Work out the finished part from the listing and answer in its coordinate system (mm). A direction names the side the tool comes from. Coordinates: 2 decimals unless noted, no trailing zeros. Use a Markdown table: item, result.
from build123d import *

# Parameters (mm, degrees)
SKIZZE2_W                            = 100
SKIZZE2_H                            = 39.364160046
AUFSATZ_LINEAR_AUSTRAGEN1_DEPTH      = 30
SCHNITT_LINEAR_AUSTRAGEN1_DEPTH      = 40
SCHNITT_LINEAR_AUSTRAGEN1_DEPTH_BACK = 40
SKIZZE10_R                           = 5
SKIZZE17_R                           = 1.4
SCHNITT_LINEAR_AUSTRAGEN2_DEPTH      = 103.710939516
SKIZZE24_R                           = 1.55
SCHNITT_LINEAR_AUSTRAGEN4_DEPTH      = 112.577493681
SKIZZE37_R                           = 0.736865544
SCHNITT_LINEAR_AUSTRAGEN9_DEPTH      = 112.577493681
SKIZZE40_R                           = 2.1
SCHNITT_LINEAR_AUSTRAGEN10_DEPTH     = 6
SKIZZE42_R                           = 0.75
SCHNITT_LINEAR_AUSTRAGEN12_DEPTH     = 10
VERRUNDUNG1_R                        = 1
SKIZZE46_R                           = 2.85
SCHNITT_LINEAR_AUSTRAGEN15_DEPTH     = 10
SCHNITT_LINEAR_START                 = -5
SCHNITT_LINEAR_AUSTRAGEN25_DEPTH     = 2.7
LINEARES_MUSTER1_COUNT               = 5
LINEARES_MUSTER1_PITCH               = 17
SPIEGELN2_COPY_1_SKETCH_R            = 2.85
SPIEGELN2_COPY_1_DEPTH               = 10
SPIEGELN2_COPY_2_SKETCH_R            = 2.85
SPIEGELN2_COPY_2_DEPTH               = 10
SPIEGELN2_COPY_3_SKETCH_R            = 2.85
SPIEGELN2_COPY_3_DEPTH               = 10
SPIEGELN2_COPY_4_SKETCH_R            = 2.85
SPIEGELN2_COPY_4_DEPTH               = 10
SPIEGELN2_START                      = -5
SPIEGELN2_COPY_5_DEPTH               = 2.7
SPIEGELN2_COPY_6_DEPTH               = 2.7
SPIEGELN2_COPY_7_DEPTH               = 2.7
SPIEGELN2_COPY_8_DEPTH               = 2.7
SKIZZE45_W                           = 15
SKIZZE45_H                           = 39.364160046
SCHNITT_LINEAR_AUSTRAGEN14_DEPTH     = 100


with BuildPart() as part:
    # Skizze2 → Aufsatz-Linear austragen1 (new body)
    with BuildSketch(Plane.XY):
        with Locations((50, 19.682080023)):
            Rectangle(SKIZZE2_W, SKIZZE2_H)
    extrude(amount=AUFSATZ_LINEAR_AUSTRAGEN1_DEPTH)

    # Skizze10 → Schnitt-Linear austragen1 (cut, two sides: drawn at the far end of the back side and taken through both)
    with BuildSketch(Plane.ZY.offset(-50).offset(-SCHNITT_LINEAR_AUSTRAGEN1_DEPTH_BACK)):
        with Locations((14.945770016, 20.027045739)):
            Circle(SKIZZE10_R)
    extrude(amount=SCHNITT_LINEAR_AUSTRAGEN1_DEPTH + SCHNITT_LINEAR_AUSTRAGEN1_DEPTH_BACK, mode=Mode.SUBTRACT)

    # Skizze17 → Schnitt-Linear austragen2 (cut, through all)
    with BuildSketch(Plane.ZY.offset(-90)):
        with Locations((14.945770016, 20.027045739)):
            Circle(SKIZZE17_R)
    schnitt_linear_austragen2 = extrude(amount=-SCHNITT_LINEAR_AUSTRAGEN2_DEPTH, mode=Mode.SUBTRACT)

    # Spiegeln1: Schnitt-Linear austragen2 across plane
    add(schnitt_linear_austragen2.mirror(Plane.ZY.offset(-50)), mode=Mode.SUBTRACT)

    # Skizze24 → Schnitt-Linear austragen4 (cut, through all)
    with BuildSketch(Plane.XY.offset(30)):
        with Locations((16, 31.364160046)):
            Circle(SKIZZE24_R)
        with Locations((33, 31.364160046)):
            Circle(SKIZZE24_R)
        with Locations((50, 31.364160046)):
            Circle(SKIZZE24_R)
        with Locations((67, 31.364160046)):
            Circle(SKIZZE24_R)
        with Locations((84, 31.364160046)):
            Circle(SKIZZE24_R)
    schnitt_linear_austragen4 = extrude(amount=-SCHNITT_LINEAR_AUSTRAGEN4_DEPTH, mode=Mode.SUBTRACT)

    # Skizze37 → Schnitt-Linear austragen9 (cut, through all)
    with BuildSketch(Plane(origin=(100, 0, 0), x_dir=(0, 0, -1), z_dir=(1, 0, 0))):
        with Locations((-18.924590299, 18.633559666)):
            Circle(SKIZZE37_R)
    extrude(amount=-SCHNITT_LINEAR_AUSTRAGEN9_DEPTH, mode=Mode.SUBTRACT)

    # Skizze40 → Schnitt-Linear austragen10 (cut)
    with BuildSketch(Plane(origin=(100, 0, 0), x_dir=(0, 0, -1), z_dir=(1, 0, 0))):
        with Locations((-18.924590299, 18.633559666)):
            Circle(SKIZZE40_R)
    extrude(amount=-SCHNITT_LINEAR_AUSTRAGEN10_DEPTH, mode=Mode.SUBTRACT)

    # Skizze42 → Schnitt-Linear austragen12 (cut)
    with BuildSketch(Plane.ZY):
        with Locations((10.86415918, 18.842582577)):
            Circle(SKIZZE42_R)
    extrude(amount=-SCHNITT_LINEAR_AUSTRAGEN12_DEPTH, mode=Mode.SUBTRACT)

    # Verrundung1
    verrundung1_edges = [part.edges().sort_by_distance(p)[0] for p in [
        (94, 18.633559666, 19.661455843),
    ]]
    fillet(verrundung1_edges, radius=VERRUNDUNG1_R)

    # Skizze46 → Schnitt-Linear austragen15 (cut)
    with BuildSketch(Plane(origin=(0, 0, 0), x_dir=(-1, 0, 0), z_dir=(0, 0, -1))):
        with Locations((-84, 31.364160046)):
            Circle(SKIZZE46_R)
    schnitt_linear_austragen15 = extrude(amount=-SCHNITT_LINEAR_AUSTRAGEN15_DEPTH, mode=Mode.SUBTRACT)

    # Skizze50 → Schnitt-Linear austragen25 (cut)
    with BuildSketch(Plane.XY.offset(30).offset(SCHNITT_LINEAR_START)):
        Polygon((81.15, 33.009608314), (81.15, 39.364160046), (86.85, 39.364160046), (86.85, 33.009608314), (86.85, 29.718711779), (84, 28.073263512), (81.15, 29.718711779), align=None)
    schnitt_linear_austragen25 = extrude(amount=-SCHNITT_LINEAR_AUSTRAGEN25_DEPTH, mode=Mode.SUBTRACT)

    # Lineares Muster1: Schnitt-Linear austragen15, Schnitt-Linear austragen25 ×5
    with Locations(*[(-i * LINEARES_MUSTER1_PITCH, 0, 0) for i in range(1, LINEARES_MUSTER1_COUNT)]):
        add(schnitt_linear_austragen15, mode=Mode.SUBTRACT)
        add(schnitt_linear_austragen25, mode=Mode.SUBTRACT)

    # Spiegeln2: Schnitt-Linear austragen15, Schnitt-Linear austragen25 across plane
    add(schnitt_linear_austragen15.mirror(Plane.ZX.offset(19.764160046)), mode=Mode.SUBTRACT)
    add(schnitt_linear_austragen25.mirror(Plane.ZX.offset(19.764160046)), mode=Mode.SUBTRACT)

    # Spiegeln2 copy 1 sketch → Spiegeln2 copy 1 (cut)
    with BuildSketch(Plane(origin=(-17, 39.528320093, 0), x_dir=(-1, 0, 0), z_dir=(0, 0, -1))):
        with Locations((-84, -31.364160046)):
            Circle(SPIEGELN2_COPY_1_SKETCH_R)
    extrude(amount=-SPIEGELN2_COPY_1_DEPTH, mode=Mode.SUBTRACT)

    # Spiegeln2 copy 2 sketch → Spiegeln2 copy 2 (cut)
    with BuildSketch(Plane(origin=(-34, 39.528320093, 0), x_dir=(-1, 0, 0), z_dir=(0, 0, -1))):
        with Locations((-84, -31.364160046)):
            Circle(SPIEGELN2_COPY_2_SKETCH_R)
    extrude(amount=-SPIEGELN2_COPY_2_DEPTH, mode=Mode.SUBTRACT)

    # Spiegeln2 copy 3 sketch → Spiegeln2 copy 3 (cut)
    with BuildSketch(Plane(origin=(-51, 39.528320093, 0), x_dir=(-1, 0, 0), z_dir=(0, 0, -1))):
        with Locations((-84, -31.364160046)):
            Circle(SPIEGELN2_COPY_3_SKETCH_R)
    extrude(amount=-SPIEGELN2_COPY_3_DEPTH, mode=Mode.SUBTRACT)

    # Spiegeln2 copy 4 sketch → Spiegeln2 copy 4 (cut)
    with BuildSketch(Plane(origin=(-68, 39.528320093, 0), x_dir=(-1, 0, 0), z_dir=(0, 0, -1))):
        with Locations((-84, -31.364160046)):
            Circle(SPIEGELN2_COPY_4_SKETCH_R)
    extrude(amount=-SPIEGELN2_COPY_4_DEPTH, mode=Mode.SUBTRACT)

    # Spiegeln2 copy 5 sketch → Spiegeln2 copy 5 (cut)
    with BuildSketch(Plane(origin=(-17, 39.528320093, 30), x_dir=(1, 0, 0), z_dir=(0, 0, 1)).offset(SPIEGELN2_START)):
        Polygon((81.15, -33.009608314), (81.15, -39.364160046), (86.85, -39.364160046), (86.85, -33.009608314), (86.85, -29.718711779), (84, -28.073263512), (81.15, -29.718711779), align=None)
    extrude(amount=-SPIEGELN2_COPY_5_DEPTH, mode=Mode.SUBTRACT)

    # Spiegeln2 copy 6 sketch → Spiegeln2 copy 6 (cut)
    with BuildSketch(Plane(origin=(-34, 39.528320093, 30), x_dir=(1, 0, 0), z_dir=(0, 0, 1)).offset(SPIEGELN2_START)):
        Polygon((81.15, -33.009608314), (81.15, -39.364160046), (86.85, -39.364160046), (86.85, -33.009608314), (86.85, -29.718711779), (84, -28.073263512), (81.15, -29.718711779), align=None)
    extrude(amount=-SPIEGELN2_COPY_6_DEPTH, mode=Mode.SUBTRACT)

    # Spiegeln2 copy 7 sketch → Spiegeln2 copy 7 (cut)
    with BuildSketch(Plane(origin=(-51, 39.528320093, 30), x_dir=(1, 0, 0), z_dir=(0, 0, 1)).offset(SPIEGELN2_START)):
        Polygon((81.15, -33.009608314), (81.15, -39.364160046), (86.85, -39.364160046), (86.85, -33.009608314), (86.85, -29.718711779), (84, -28.073263512), (81.15, -29.718711779), align=None)
    extrude(amount=-SPIEGELN2_COPY_7_DEPTH, mode=Mode.SUBTRACT)

    # Spiegeln2 copy 8 sketch → Spiegeln2 copy 8 (cut)
    with BuildSketch(Plane(origin=(-68, 39.528320093, 30), x_dir=(1, 0, 0), z_dir=(0, 0, 1)).offset(SPIEGELN2_START)):
        Polygon((81.15, -33.009608314), (81.15, -39.364160046), (86.85, -39.364160046), (86.85, -33.009608314), (86.85, -29.718711779), (84, -28.073263512), (81.15, -29.718711779), align=None)
    extrude(amount=-SPIEGELN2_COPY_8_DEPTH, mode=Mode.SUBTRACT)

    # Spiegeln3: Schnitt-Linear austragen4 across plane
    add(schnitt_linear_austragen4.mirror(Plane.ZX.offset(19.764160046)), mode=Mode.SUBTRACT)

    # Skizze45 → Schnitt-Linear austragen14 (cut)
    with BuildSketch(Plane(origin=(100, 0, 0), x_dir=(0, 0, -1), z_dir=(1, 0, 0))):
        with Locations((-7.5, 19.682080023)):
            Rectangle(SKIZZE45_W, SKIZZE45_H)
    extrude(amount=-SCHNITT_LINEAR_AUSTRAGEN14_DEPTH, mode=Mode.SUBTRACT)


solid = part.part
(1) Given P1, Ø0.8, axis at x = 84, z = 24.5, coming from the +Y side; P2, Ø1.3, axis at x = 14.5, z = 23, coming from the +Y side, each flat-ended and moving along its own axis, determine where each tip first touches the part or whether it passes through.
Conclusion:
| item | result |
|---|---|
| P1 | y = 28.3 |
| P2 | y = 29.31 |
(2) Which of the six approach directions +Z, -Z, +X, -X, +Y, -Y give full straight-line access (tool end or side, diameter ignored) to faces 4 (the flat face through (86.85, 5, 24)), 5 (the flat face through (90, 20, 17)), 6 (the flat face through (50, 35, 25))?
Conclusion:
| item | result |
|---|---|
| face 4 | none |
| face 5 | -Z |
| face 6 | +Y |
(3) Straight lines are drawn through the part: L1, parallel to X at y = 8, z = 20.25; L2, parallel to X at y = 36, z = 24.25; L3, parallel to Z at x = 83.5, y = 36.5. For each, find the intervals that lie inside material, in ascending order.
Conclusion:
| item | result |
|---|---|
| L1 | 0 to 14.46, 17.54 to 31.46, 34.54 to 48.46, 51.54 to 65.46, 68.54 to 82.46, 85.54 to 100 |
| L2 | 0 to 13.15, 18.85 to 30.15, 35.85 to 47.15, 52.85 to 64.15, 69.85 to 81.15, 86.85 to 100 |
| L3 | 15 to 22.3, 25 to 30 |
(4) Determine the mould class of faces 1 (the flat face through (65.59, 10.64, 23.67)), 2 (the flat face through (48.595, 28.884, 23.669)), 3 (the flat face through (51, 34, 15)) for opening direction Y: pulls with the +Y half, pulls with the -Y half, needs draft (parallel to the pull), parting line crosses it, or undercut.
Conclusion:
| item | result |
|---|---|
| face 1 | undercut |
| face 2 | pulls with the +Y half |
| face 3 | needs draft |
(5) A cutting plane is placed at A-A (z = 27). Give the number of separate pieces and of enclosed holes in the cut face, then the cut area to 3 significant figures.
Conclusion:
| item | result |
|---|---|
| separate pieces | 1 |
| enclosed holes | 10 |
| area | 3,860 mm2 |
